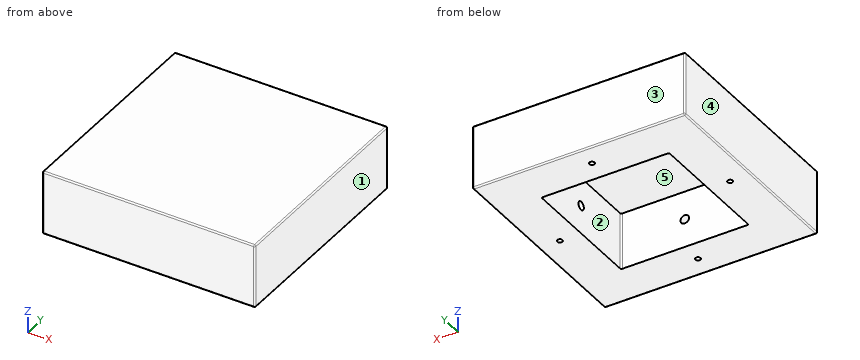
from build123d import *

# Parameters (mm, degrees)
SKETCH1_W           = 150
SKETCH1_H           = 150
BOSS_EXTRUDE1_DEPTH = 45
SKETCH2_W           = 90
SKETCH2_H           = 90
CUT_EXTRUDE1_DEPTH  = 40
SKETCH6_R           = 1.8
CUT_EXTRUDE2_DEPTH  = 20
CIRPATTERN1_COUNT   = 2
CIRPATTERN1_ANGLE   = 90
SKETCH8_R           = 3
CUT_EXTRUDE4_DEPTH  = 17
CIRPATTERN2_COUNT   = 4
FILLET1_R           = 1
FILLET2_R           = 1


with BuildPart() as part:
    # Sketch1 → Boss-Extrude1 (new body)
    with BuildSketch(Plane.XY):
        with Locations((75, 75)):
            Rectangle(SKETCH1_W, SKETCH1_H)
    extrude(amount=BOSS_EXTRUDE1_DEPTH)

    # Sketch2 → Cut-Extrude1 (cut)
    with BuildSketch(Plane.XY):
        with Locations((75, 75)):
            Rectangle(SKETCH2_W, SKETCH2_H)
    extrude(amount=CUT_EXTRUDE1_DEPTH, mode=Mode.SUBTRACT)

    # Sketch6 → Cut-Extrude2 (cut)
    with BuildSketch(Plane(origin=(0, 0, 0), x_dir=(-1, 0, 0), z_dir=(0, 0, -1))):
        with Locations((-135, 75)):
            Circle(SKETCH6_R)
        with Locations((-15, 75)):
            Circle(SKETCH6_R)
    cut_extrude2 = extrude(amount=-CUT_EXTRUDE2_DEPTH, mode=Mode.SUBTRACT)

    # CirPattern1: Cut-Extrude2 ×2 about axis
    cirpattern1_axis = Axis((75, 75, 0), (0, 0, -1))
    for i in range(1, CIRPATTERN1_COUNT):
        add(cut_extrude2.rotate(cirpattern1_axis, i * CIRPATTERN1_ANGLE / (CIRPATTERN1_COUNT - 1)), mode=Mode.SUBTRACT)

    # Sketch8 → Cut-Extrude4 (cut)
    with BuildSketch(Plane(origin=(120, 0, 0), x_dir=(0, 0, -1), z_dir=(1, 0, 0))):
        with Locations(Location((-20, 75, 0), (0, 0, 90))):
            Circle(SKETCH8_R)
    cut_extrude4 = extrude(amount=CUT_EXTRUDE4_DEPTH, mode=Mode.SUBTRACT)

    # CirPattern2: Cut-Extrude4 ×4 about axis
    cirpattern2_axis = Axis((75, 75, 0), (0, 0, 1))
    for i in range(1, CIRPATTERN2_COUNT):
        add(cut_extrude4.rotate(cirpattern2_axis, i * 360 / CIRPATTERN2_COUNT), mode=Mode.SUBTRACT)

    # Fillet1
    fillet1_edges = [part.edges().sort_by_distance(p)[0] for p in [
        (75, 150, 45),
        (0, 75, 45),
        (75, 0, 45),
        (0, 75, 0),
        (75, 150, 0),
        (150, 75, 0),
        (75, 0, 0),
        (0, 0, 22.5),
        (0, 150, 22.5),
        (150, 150, 22.5),
        (150, 0, 22.5),
        (150, 75, 45),
    ]]
    fillet(fillet1_edges, radius=FILLET1_R)

    # Fillet2
    fillet2_edges = [part.edges().sort_by_distance(p)[0] for p in [
        (120, 30, 20),
        (120, 120, 20),
        (30, 120, 20),
        (30, 30, 20),
    ]]
    fillet(fillet2_edges, radius=FILLET2_R)


solid = part.part
Can you work these out from the model? Positions are in its coordinate system, mm. Face numbers are marked on the shaded views. A direction names the side the tool comes from. Coordinates: 2 decimals unless noted, no trailing zeros. Loops run counter-clockwise (first coordinate to the right, second up) from the corner with the lowest first, then second, coordinate; pieces in that order, holes last. Notation, with made-up numbers: (-13, -36) - (26, -36) arc R26 cw to (26, -2) - close; hole circle Ø11 at (77, -13). An arc over 180 degrees is marked (long way). Put each result on its own line as item: value. Start each with the question number.
Item 1: For pin 1 (2 mm diameter, centred on x = 75, y = 135, fed in from -Z); pin 2 (4.5 mm diameter, centred on x = 75, y = 15, fed in from -Z), each with a flat end and sliding along its axis, tell me the tip position at first contact or that it passes through.
Item 2: If we mould it in two halves opening along X, with no side actions, what happens to the marked faces 1, 2 and 3? For each: +X half, -X half, draft (parallel to the pull), parting line (faces both ways), or undercut.
Item 3: If I drill on line 1 along X through (y, z) = (75, 12); line 2 along Y through (x, z) = (42.5, 29), over which ranges is the centre line in solid material (lowest first)?
Item 4: Which directions (+Z, -Z, +X, -X, +Y, -Y) give clear straight access to the entire face, cutting with the end or side of a thin tool? Please do the marked faces 4 and 5.
Item 5: Suppose I cut it at A-A (y = 75). Please give me the cut outline in (x, z).
Item 6: Suppose I cut it at D-D (y = 97). Please give me the cut outline in (x, z), and give its area (3 significant figures).
Here are the results:
1. pin 1: z = 22.83
1. pin 2: z = 0
2. face 1: +X half
2. face 2: undercut
2. face 3: draft
3. line 1: 0 to 13.2, 16.8 to 30, 120 to 133.2, 136.8 to 150
3. line 2: 0 to 30, 120 to 150
4. face 4: +Z, -Z, -X, +Y, -Y
4. face 5: -Z
5. outline: (0, 1) arc R1 ccw to (1, 0) - (13.2, 0) - (13.2, 17) - (13, 17) - (13, 23) - (30, 23) - (30, 40) - (120, 40) - (120, 23) - (137, 23) - (137, 17) - (136.8, 17) - (136.8, 0) - (149, 0) arc R1 ccw to (150, 1) - (150, 44) arc R1 ccw to (149, 45) - (1, 45) arc R1 ccw to (0, 44) - close; (16.8, 0) - (30, 0) - (30, 17) - (16.8, 17) - close; (120, 0) - (133.2, 0) - (133.2, 17) - (120, 17) - close
6. outline: (0, 1) arc R1 ccw to (1, 0) - (30, 0) - (30, 40) - (120, 40) - (120, 0) - (149, 0) arc R1 ccw to (150, 1) - (150, 44) arc R1 ccw to (149, 45) - (1, 45) arc R1 ccw to (0, 44) - close
6. area: 3,150 mm²
